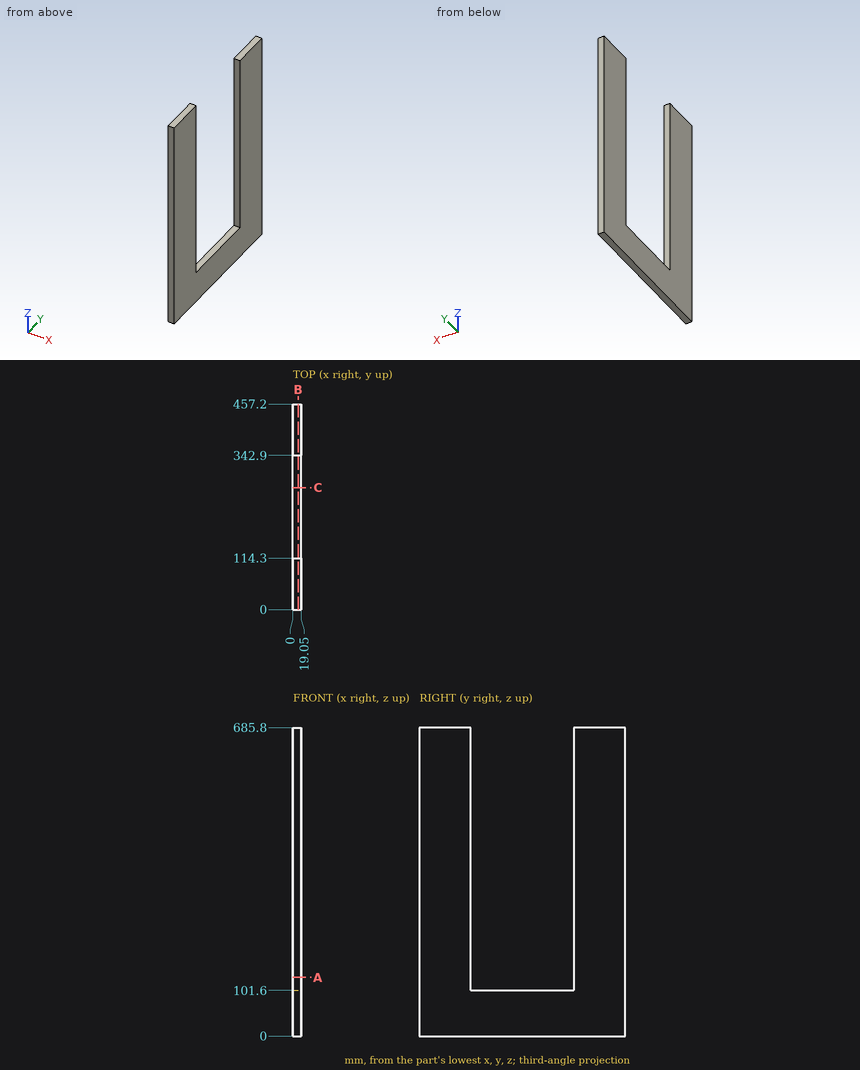
Study the drawing (mm; zero at the part's minimum x, y, z) and answer. Round coordinates to 2 decimals unless told otherwise and drop trailing zeros. Write each loop counter-clockwise with the first axis right and the second up, starting at its lowest first coordinate (ties: lowest second). Pieces come first, ordered by that corner, then holes.
1) A cutting plane is placed at A-A on z = 130.5. Determine the outline of the cut face in (x, y), and give its area (3 significant figures).
2) Consider probe 1 along Y at (x, z) = (3.25, 219); probe 2 along Z at (x, y) = (5.75, 153). Determine where each line is inside the solid, lowest interval first.
3) A cutting plane is placed at B-B on x = 11.5. Determine the outline of the cut face in (y, z).
4) A flat-ended cylindrical pin translates along its axis: P1, Ø5.5, axis at x = 13, y = 180.5, coming from the +Z side. Find the tip coordinate at first contact, or state that the pin passes through.
5) A cutting plane is placed at C-C on y = 271.5. Determine the outline of the cut face in (x, z).
Entries:
1. outline: (0, 0) - (19.05, 0) - (19.05, 114.3) - (0, 114.3) - close; (0, 342.9) - (19.05, 342.9) - (19.05, 457.2) - (0, 457.2) - close
1. area: 4,350 mm2
2. probe 1: y = 0 to 114.3, 342.9 to 457.2
2. probe 2: z = 0 to 101.6
3. outline: (0, 0) - (457.2, 0) - (457.2, 685.8) - (342.9, 685.8) - (342.9, 101.6) - (114.3, 101.6) - (114.3, 685.8) - (0, 685.8) - close
4. P1: stops at z = 101.6
5. outline: (0, 0) - (19.05, 0) - (19.05, 101.6) - (0, 101.6) - close
